from build123d import *

# Parameters (mm, degrees)
F0_R     = 18.8
F0_R_2   = 4.25
F0_R_3   = 3.5
F1_DEPTH = 1.8
F2_R     = 0.5


with BuildPart() as f1:
    # F0 (on Top) → F1 (new body)
    with BuildSketch(Plane.XY):
        Circle(F0_R)
        with Locations((-3.476441, -10.699386)):
            Circle(F0_R_2, mode=Mode.SUBTRACT)
        with BuildLine():
            Line((-3.485354, -4.254681), (-3.712655, -4.95424))
            ThreePointArc((-3.712655, -4.95424), (-8.945016, -8.922538), (-7.044454, -15.208464))
            Line((-7.044454, -15.208464), (-7.11892, -15.437648))
            ThreePointArc((-7.11892, -15.437648), (-13.753289, -9.992349), (-16.881943, -2))
            Line((-16.881943, -2), (-16.640965, -2))
            ThreePointArc((-16.640965, -2), (-11.25, -5.75), (-5.859035, -2))
            Line((-5.859035, -2), (-5.123475, -2))
            ThreePointArc((-5.123475, -2), (-4.449593, -3.232819), (-3.485354, -4.254681))
        make_face(mode=Mode.SUBTRACT)
        with BuildLine():
            ThreePointArc((12.482208, -11.540991), (5.253289, -16.167961), (-3.314694, -16.673716))
            Line((-3.314694, -16.673716), (-3.240228, -16.444532))
            ThreePointArc((-3.240228, -16.444532), (1.992134, -12.476234), (0.091572, -6.190308))
            Line((0.091572, -6.190308), (0.318872, -5.490749))
            ThreePointArc((0.318872, -5.490749), (1.699593, -5.230811), (2.969408, -4.629537))
            Line((2.969408, -4.629537), (3.564489, -5.061889))
            ThreePointArc((3.564489, -5.061889), (5.721676, -11.264432), (12.287253, -11.399348))
            Line((12.287253, -11.399348), (12.482208, -11.540991))
        make_face(mode=Mode.SUBTRACT)
        with Locations((9.101441, -6.612584)):
            Circle(F0_R_2, mode=Mode.SUBTRACT)
        with Locations((-11.25, 0)):
            Circle(F0_R_2, mode=Mode.SUBTRACT)
        with BuildLine():
            Line((-3.712655, 4.95424), (-3.485354, 4.254681))
            ThreePointArc((-3.485354, 4.254681), (-4.449593, 3.232819), (-5.123475, 2))
            Line((-5.123475, 2), (-5.859035, 2))
            ThreePointArc((-5.859035, 2), (-11.25, 5.75), (-16.640965, 2))
            Line((-16.640965, 2), (-16.881943, 2))
            ThreePointArc((-16.881943, 2), (-13.753289, 9.992349), (-7.11892, 15.437648))
            Line((-7.11892, 15.437648), (-7.044454, 15.208464))
            ThreePointArc((-7.044454, 15.208464), (-8.945016, 8.922538), (-3.712655, 4.95424))
        make_face(mode=Mode.SUBTRACT)
        with Locations((-3.476441, 10.699386)):
            Circle(F0_R_2, mode=Mode.SUBTRACT)
        Circle(F0_R_3, mode=Mode.SUBTRACT)
        with Locations((9.101441, 6.612584)):
            Circle(F0_R_2, mode=Mode.SUBTRACT)
        with BuildLine():
            Line((14.833349, -8.304923), (14.638394, -8.16328))
            ThreePointArc((14.638394, -8.16328), (12.481206, -1.960736), (5.91563, -1.825821))
            Line((5.91563, -1.825821), (5.320549, -1.393469))
            ThreePointArc((5.320549, -1.393469), (5.5, 0), (5.320549, 1.393469))
            Line((5.320549, 1.393469), (5.91563, 1.825821))
            ThreePointArc((5.91563, 1.825821), (12.481206, 1.960736), (14.638394, 8.16328))
            Line((14.638394, 8.16328), (14.833349, 8.304923))
            ThreePointArc((14.833349, 8.304923), (17, 0), (14.833349, -8.304923))
        make_face(mode=Mode.SUBTRACT)
        with BuildLine():
            ThreePointArc((-3.314694, 16.673716), (5.253289, 16.167961), (12.482208, 11.540991))
            Line((12.482208, 11.540991), (12.287253, 11.399348))
            ThreePointArc((12.287253, 11.399348), (5.721676, 11.264432), (3.564489, 5.061889))
            Line((3.564489, 5.061889), (2.969408, 4.629537))
            ThreePointArc((2.969408, 4.629537), (1.699593, 5.230811), (0.318872, 5.490749))
            Line((0.318872, 5.490749), (0.091572, 6.190308))
            ThreePointArc((0.091572, 6.190308), (1.992134, 12.476234), (-3.240228, 16.444532))
            Line((-3.240228, 16.444532), (-3.314694, 16.673716))
        make_face(mode=Mode.SUBTRACT)
    extrude(amount=F1_DEPTH)

    # F2
    f2_edges = [f1.edges().sort_by_distance(p)[0] for p in [
        (-18.8, 0, 1.8),
        (-18.8, 0, 0),
    ]]
    fillet(f2_edges, radius=F2_R)


solid = f1.part
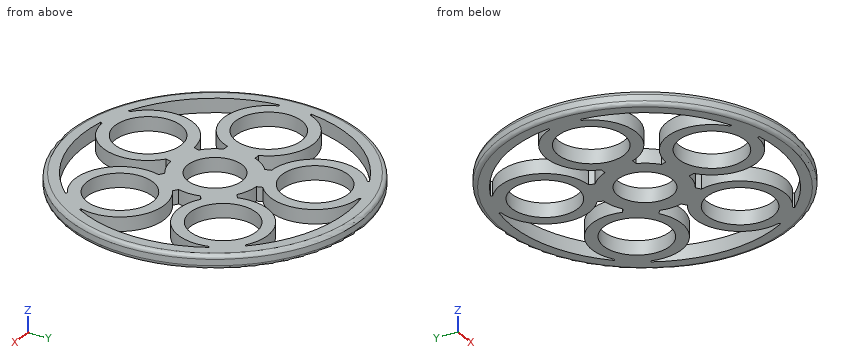
Here's how the part is built. I have some questions about the finished solid (model axes, mm). Round coordinates to 2 decimals unless told otherwise and drop trailing zeros. Order: outer loops, then holes, each group sorted by start corner. A loop starts at its lowest first (then second) coordinate and runs counter-clockwise, first axis right, second up. Notation, with made-up numbers: M -28.5,-37.5 L -23.5,-37.5 A23 cw -23.5,-8.5 Z; hole C 3.5,44 d10. An arc over 180 degrees is marked long. One line per question, with ' | ' between items.
1) I'm going to push flat-ended pins straight in: pin 1 Ø0.8 at (x, z) = (-5.5, 0.5) entering from -Y (3 decimals); pin 2 Ø1 at (y, z) = (-13, 1.5) entering from +X. Where does each tip first touch, or does it pass through?
Checked values:
pin 1: stops at y = -18.095 | pin 2: stops at x = 14.02
2) Imagine slicing it at B-B, the plane y = 9. Count the separate pieces of the cut face and the enclosed holes in it, plus the area to 3 significant figures.
Checked values:
separate pieces: 5 | enclosed holes: 0 | area: 19.3 mm²
3) Imagine slicing it at A-A, the plane y = 0. Write out the boundary of the cut face in (x, z), plus the area to 3 significant figures.
Checked values:
outline: M -18.8,0.5 A0.5 ccw -18.3,0 L -15.5,0 L -15.5,1.8 L -18.3,1.8 A0.5 ccw -18.8,1.3 Z; M -7,0 L -3.5,0 L -3.5,1.8 L -7,1.8 Z; M 3.5,0 L 5.5,0 L 5.5,1.8 L 3.5,1.8 Z; M 17,0 L 18.3,0 A0.5 ccw 18.8,0.5 L 18.8,1.3 A0.5 ccw 18.3,1.8 L 17,1.8 Z | area: 18.9 mm²
4) I need wall thicknesses on line 1 (Y direction, x = -5, z = 0.85); line 2 (X direction, y = 8, z = 1.6); line 3 (Y direction, x = -6, z = 1.15). Which ranges of each line are inside material? Lowest first, please.
Checked values:
line 1: y = -18.12 to -14.67, -6.73 to -5.15, -2.29 to 2.29, 5.15 to 6.73, 14.67 to 18.12 | line 2: x = -16.9 to -15, -8.55 to -6.76, -0.19 to 1.6, 3.52 to 5.08, 13.12 to 14.68, 15 to 16.9 | line 3: y = -17.82 to -14.12, -7.28 to -5.53, -2.35 to 2.35, 5.53 to 7.28, 14.12 to 17.82
